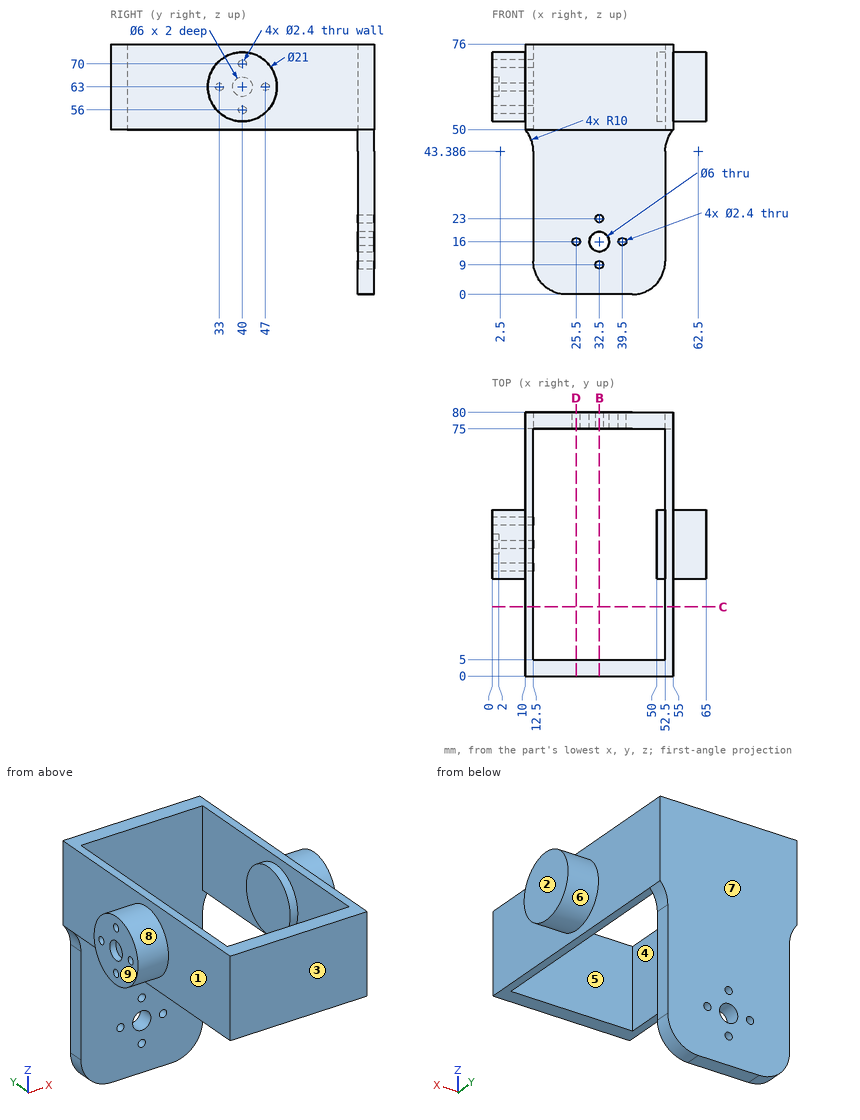
Print and shaded views of the part. All mm, measured from the part's lowest x, y and z. A direction names the side the tool comes from. Round coordinates to 2 decimals unless told otherwise and drop trailing zeros. Write each loop counter-clockwise with the first axis right and the second up, starting at its lowest first coordinate (ties: lowest second). Pieces come first, ordered by that corner, then holes. Notation, with made-up numbers: (85, -0.5) -> (128, -0.5) arc R9 ccw to (128, 10.5) -> close; hole circle Ø7 at (66.5, 27.25). An arc over 180 degrees is marked (long way). Answer in a Markdown table with one row per item. Add a question column.
Item 1: Drill centre lines: line 1 (Y direction, x = 7.75, z = 63); line 2 (X direction, y = 76, z = 16); line 3 (Y direction, x = 35.5, z = 54). Where is each one in solid material? Low to high. Write a range as from..to.
Item 2: Saw through at C-C, the plane y = 21. Write the cut outline in (x, z), then the cut area to 3 significant figures.
Item 3: Mould opens along X. For the marked faces 1, 2, 3 and 4 say: pulls with the +X half, pulls with the -X half, needs draft (parallel to the pull), parting line crosses it, or undercut.
Item 4: Drop flat-ended pins along their axis: pin 1 Ø1.4 at (y, z) = (33, 63) entering from -X; pin 2 Ø4 at (y, z) = (47, 63) entering from -X; pin 3 Ø3 at (x, z) = (25.5, 16) entering from -Y; pin 4 Ø3.5 at (y, z) = (40, 63) entering from -X. Give the stop position or say it passes through.
Item 5: Which spindle directions (+Z, -Z, +X, -X, +Y, -Y) get a long thin tool onto all of the face, cutting with end or side? Do the marked faces 5, 6, 7, 8 and 9. Say none if no direction does.
Item 6: Saw through at D-D, the plane x = 25.5. Write the cut outline in (y, z).
Item 7: Saw through at B-B, the plane x = 32.5. Write the cut outline in (y, z), then the cut area to 3 significant figures.
Findings below:
| question | item | result |
|---|---|---|
| 1 | line 1 | y = 29.5..31.8, 34.2..45.8, 48.2..50.5 |
| 1 | line 2 | x = 12.5..24.3, 26.7..29.5, 35.5..38.3, 40.7..52.5 |
| 1 | line 3 | y = 0..5, 75..80 |
| 2 | outline | (10, 50) -> (12.5, 50) -> (12.5, 76) -> (10, 76) -> close; (52.5, 50) -> (55, 50) -> (55, 76) -> (52.5, 76) -> close |
| 2 | area | 130 mm^2 |
| 3 | face 1 | pulls with the -X half |
| 3 | face 2 | pulls with the +X half |
| 3 | face 3 | needs draft |
| 3 | face 4 | undercut |
| 4 | pin 1 | stops at x = 50 |
| 4 | pin 2 | stops at x = 0 |
| 4 | pin 3 | stops at y = 75 |
| 4 | pin 4 | stops at x = 2 |
| 5 | face 5 | +Z, -Z |
| 5 | face 6 | +X |
| 5 | face 7 | +Z, -Z, +X, -X, +Y |
| 5 | face 8 | -X |
| 5 | face 9 | +Z, -Z, -X, +Y, -Y |
| 6 | outline | (0, 50) -> (5, 50) -> (5, 76) -> (0, 76) -> close; (75, 0) -> (80, 0) -> (80, 14.8) -> (75, 14.8) -> close; (75, 17.2) -> (80, 17.2) -> (80, 76) -> (75, 76) -> close |
| 7 | outline | (0, 50) -> (5, 50) -> (5, 76) -> (0, 76) -> close; (75, 0) -> (80, 0) -> (80, 7.8) -> (75, 7.8) -> close; (75, 10.2) -> (80, 10.2) -> (80, 13) -> (75, 13) -> close; (75, 19) -> (80, 19) -> (80, 21.8) -> (75, 21.8) -> close; (75, 24.2) -> (80, 24.2) -> (80, 76) -> (75, 76) -> close |
| 7 | area | 456 mm^2 |
